Check sheet for the modelled part. Datum: model origin and axes. Units: mm. Face numbers are marked on the shaded views. A direction names the side the tool comes from. Round coordinates to 2 decimals unless told otherwise and drop trailing zeros. Order: outer loops, then holes, each group sorted by start corner. A loop starts at its lowest first (then second) coordinate and runs counter-clockwise, first axis right, second up. Notation, with made-up numbers: (13, 0) -> (65, 0) arc R30 cw to (65, 31) -> close; hole circle Ø6 at (-13.5, 60). An arc over 180 degrees is marked (long way). Answer in a Markdown table with one row per item. Add a question column.
1. Sectioned sample at A-A, the plane z = 56. Record the boundary of the cut face in (x, y), then the cut area to 3 significant figures.
2. Material ranges on L1, parallel to Y at x = 0, z = 2.9; L2, parallel to Y at x = 1.5, z = 98; L3, parallel to Y at x = 53, z = 34, recorded low to high. Write a range as from..to.
3. Access from +Z, -Z, +X, -X, +Y, -Y to the whole of each face (thin tool, end or side, straight path). Record for the marked faces 1 and 2.
4. Depth check by flat-ended pin: P1, Ø2, axis at x = -12, y = -3.5, coming from the -Z side; P2, Ø1.5, axis at x = 9, z = 141, coming from the +Y side; P3, Ø12, axis at y = -41.5, z = 28, coming from the -X side. Enter the tip coordinate at first touch or a pass-through.
```python
from build123d import *


with BuildPart() as part:
    # Sketch001 → Revolution (revolve)
    with BuildSketch(Plane.XZ):
        with BuildLine():
            Line((65, 0), (65, 5))
            Line((65, 5), (63, 5))
            Line((63, 5), (63, 2))
            Line((63, 2), (61, 2))
            Line((61, 2), (61, 132))
            add(Edge.make_bspline(
                [(0, 200), (46.719524, 200.024536), (61, 132), (61, 132)],
                knots=[0, 0, 0, 0, 1, 1, 1, 1], degree=3))
            Line((0, 200), (0, 198))
            add(Edge.make_bspline(
                [(0, 198), (43.327412, 190.171173), (59, 130), (59, 130)],
                knots=[0, 0, 0, 0, 1, 1, 1, 1], degree=3))
            Line((59, 130), (59, 0))
            Line((59, 0), (65, 0))
        make_face()
    revolve(axis=Axis((0, 0, 0), (0, 0, 1)))


solid = part.part
```
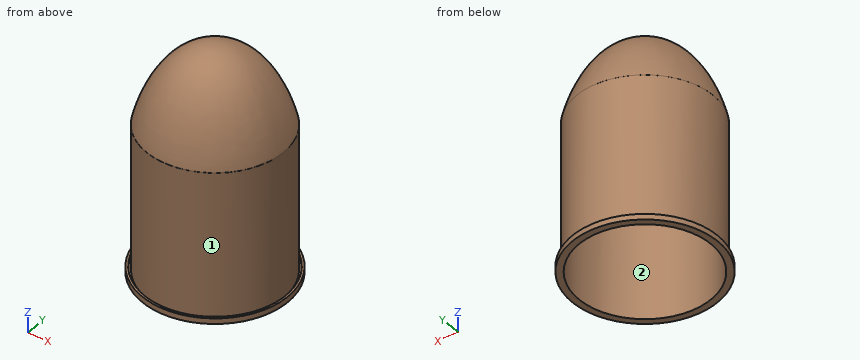
Answer key:
| question | item | result |
|---|---|---|
| 1 | outline | circle Ø122 at (0, 0); hole circle Ø118 at (0, 0) |
| 1 | area | 754 mm² |
| 2 | L1 | y = -65..-63, -61..-59, 59..61, 63..65 |
| 2 | L2 | y = -60.98..-58.98, 58.98..60.98 |
| 2 | L3 | y = -30.2..-25.92, 25.92..30.2 |
| 3 | face 1 | +Z |
| 3 | face 2 | -Z |
| 4 | P1 | stops at z = 193.57 |
| 4 | P2 | stops at y = 58.12 |
| 4 | P3 | stops at x = -49.61 |
